Here's how the part is built. I have some questions about the finished solid (model axes, mm). Face numbers are marked on the shaded views. A direction names the side the tool comes from. Round coordinates to 2 decimals unless told otherwise and drop trailing zeros. Order: outer loops, then holes, each group sorted by start corner. A loop starts at its lowest first (then second) coordinate and runs counter-clockwise, first axis right, second up. Notation, with made-up numbers: M 84,56 L 97,56 A38 ccw 97,95 Z; hole C 64.5,5.5 d2. An arc over 180 degrees is marked long. Answer as CSV lines item,"result". Start each with the question number.
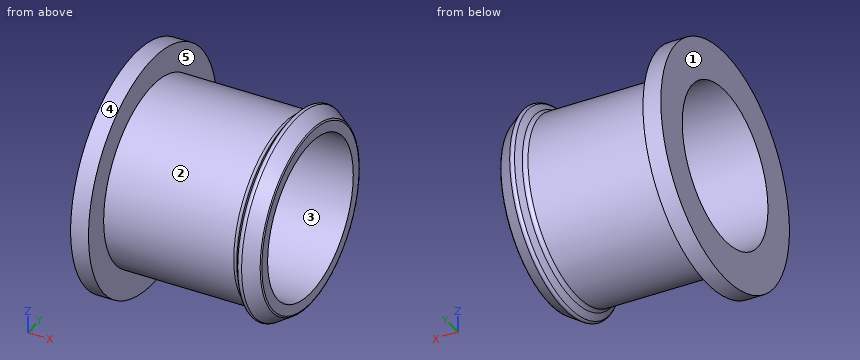
```python
from build123d import *


with BuildPart() as f1:
    # F0 (on Top) → F1 (revolve)
    with BuildSketch(Plane.XY):
        with BuildLine():
            Line((1.0795, 14.2875), (-1.0795, 14.2875))
            Line((-1.0795, 14.2875), (-1.0795, 9.525))
            Line((-1.0795, 9.525), (1.0795, 9.525))
            Line((1.0795, 9.525), (20.1295, 9.525))
            Line((20.1295, 9.525), (20.1295, 10.797701))
            ThreePointArc((20.1295, 10.797701), (20.10202, 10.907294), (20.026081, 10.990955))
            Line((20.026081, 10.990955), (18.378363, 12.089584))
            ThreePointArc((18.378363, 12.089584), (18.092305, 12.146192), (17.850004, 11.983947))
            Line((17.850004, 11.983947), (17.330457, 11.204732))
            ThreePointArc((17.330457, 11.204732), (17.101739, 10.997127), (16.802127, 10.922))
            Line((16.802127, 10.922), (1.0795, 10.922))
            Line((1.0795, 10.922), (1.0795, 14.2875))
        make_face()
    revolve(axis=Axis((9.354087, 0, 0), (1, 0, 0)))


solid = f1.part
```
Item 1: If we section it at C-C on x = 8.5: Please give me the cut outline in (y, z) (3 decimals), and give its area (3 significant figures).
Item 2: For P1, Ø1.5, axis at x = 13.5, y = -10.5, coming from the +Z side; P2, Ø1.5, axis at x = 1, y = 1, coming from the +Z side; P3, Ø4, axis at x = 11, y = -0.5, coming from the +Z side; P4, Ø11.5, axis at y = 0, z = 0, coming from the -X side, each with a flat end and sliding along its axis, tell me the tip position at first contact or that it passes through.
Item 3: If I drill on line 1 along Z through (x, y) = (12.75, 0) (3 decimals); line 2 along X through (y, z) = (10.25, -9); line 3 along Z through (x, y) = (13.25, -5), over which ranges is the centre line in solid material (lowest first)?
Item 4: Which directions (+Z, -Z, +X, -X, +Y, -Y) give clear straight access to the entire face, cutting with the end or side of a thin tool? Please do the marked faces 1 and 2.
Item 5: We'd pull the mould along Y, two halves only. Please class the marked faces 3, 4 and 5: pulls with the +Y half, pulls with the -Y half, needs draft (parallel to the pull), parting line crosses it, or undercut.
Geometry says:
1,outline,"C 0,0 d21.844; hole C 0,0 d19.05"
1,area,"89.7 mm²"
2,P1,"z = 4.92"
2,P2,"z = 14.29"
2,P3,"z = 10.92"
2,P4,"through"
3,line 1,"-10.922 to -9.525, 9.525 to 10.922"
3,line 2,"-1.08 to 1.08"
3,line 3,"-9.71 to -8.11, 8.11 to 9.71"
4,face 1,"+Z, -Z, -X, +Y, -Y"
4,face 2,"none"
5,face 3,"undercut"
5,face 4,"parting line crosses it"
5,face 5,"needs draft"
